CAD build for the part. Positions are in the model's coordinates, mm. Coordinates: 2 decimals unless noted, no trailing zeros. Write each loop counter-clockwise with the first axis right and the second up, starting at its lowest first coordinate (ties: lowest second). Pieces come first, ordered by that corner, then holes. Notation, with made-up numbers: (54, 62) - (112, 62) arc R8 ccw to (112, 77) - close; hole circle Ø9 at (19.25, 76). An arc over 180 degrees is marked (long way). Answer in a Markdown table with one row per item. Add a question column.
Q1. Band-saw the part on C-C (x = 116). List the corners of the cut face in (y, z).
Q2. Band-saw the part on B-B (y = 6). List the corners of the cut face in (x, z), and give its area (3 significant figures).
Q3. Pin check, flat tips, straight feed: pin 1 (3.5 mm diameter, centred on x = 4, y = 6, fed in from -Z); pin 2 (7 mm diameter, centred on x = 116, y = 6, fed in from +Z). Stop position of each tip, or through.
Q4. Band-saw the part on A-A (z = 1.35). List the corners of the cut face in (x, y).
Q5. Drill centre lines: line 1 along X through (y, z) = (6, 1.9); line 2 along X through (y, z) = (6.5, 4.2); line 3 along Y through (x, z) = (4, 0.85). Where is each one in solid material? Low to high. Write a range as from..to.
Q6. Band-saw the part on D-D (x = 89.5). List the corners of the cut face in (y, z), and give its area (3 significant figures).
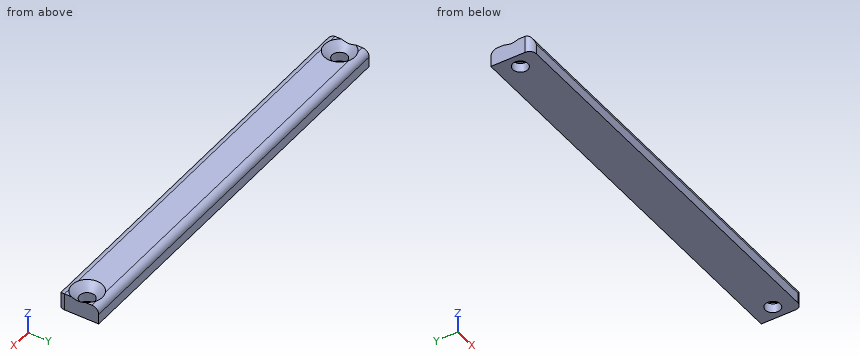
```python
from build123d import *

# Parameters (mm, degrees)
F0_W           = 120
F0_H           = 12
F1_DEPTH       = 5
F3_D           = 4.4
F3_DEPTH       = 18
F3_CSINK_D     = 8.96
F3_CSINK_ANGLE = 90
F3_TIP         = 1.3218933619
F4_T1_DEPTH    = 130
F4_T3_DEPTH    = 15


# Not quite as in the source:
# - a fillet or chamfer that OpenCascade refuses, or shapes differently, is made with other operations: its cross-section is extruded or revolved along the edge and cut away or added


with BuildPart() as f1:
    # F0 (on Top) → F1 (new body)
    with BuildSketch(Plane.XY):
        with Locations((60, 6)):
            Rectangle(F0_W, F0_H)
    extrude(amount=F1_DEPTH)

    # F3
    with Locations(Plane.XY.offset(5)):
        with Locations((4, 6), (116, 6)):
            CounterSinkHole(F3_D / 2, F3_CSINK_D / 2, depth=F3_DEPTH, counter_sink_angle=F3_CSINK_ANGLE)
            with Locations((0, 0, -(F3_DEPTH + F3_TIP / 2))):  # 118° drill point
                Cone(0, F3_D / 2, F3_TIP, mode=Mode.SUBTRACT)

    # F4: fillet of radius 2 on 4 edges, made by hand

    # F4_s2 → F4_t1 (cut)
    with BuildSketch(Plane.YZ.offset(-5)):
        with BuildLine():
            ThreePointArc((0, 3), (0.5857864376, 4.4142135624), (2, 5))
            Line((2, 5), (0, 5))
            Line((0, 5), (0, 3))
        make_face()
        with BuildLine():
            ThreePointArc((10, 5), (11.4142135624, 4.4142135624), (12, 3))
            Line((12, 3), (12, 5))
            Line((12, 5), (10, 5))
        make_face()
    extrude(amount=F4_T1_DEPTH, mode=Mode.SUBTRACT)

    # F4_s4 → F4_t3 (cut)
    with BuildSketch(Plane.XY.offset(-5)):
        with BuildLine():
            ThreePointArc((0, 2), (0.5857864376, 0.5857864376), (2, 0))
            Line((2, 0), (0, 0))
            Line((0, 0), (0, 2))
        make_face()
        with BuildLine():
            ThreePointArc((118, 0), (119.4142135624, 0.5857864376), (120, 2))
            Line((120, 2), (120, 0))
            Line((120, 0), (118, 0))
        make_face()
    extrude(amount=F4_T3_DEPTH, mode=Mode.SUBTRACT)


solid = f1.part
```
Checked values:
| question | item | result |
|---|---|---|
| 1 | outline | (0, 0) - (3.8, 0) - (3.8, 2.72) - (1.57, 4.95) arc R2 ccw to (0, 3) - close; (8.2, 0) - (12, 0) - (12, 3) arc R2 ccw to (10.43, 4.95) - (8.2, 2.72) - close |
| 2 | outline | (0, 0) - (1.8, 0) - (1.8, 2.72) - (0, 4.52) - close; (6.2, 0) - (113.8, 0) - (113.8, 2.72) - (111.52, 5) - (8.48, 5) - (6.2, 2.72) - close; (118.2, 0) - (120, 0) - (120, 4.52) - (118.2, 2.72) - close |
| 2 | area | 546 mm² |
| 3 | pin 1 | passes through |
| 3 | pin 2 | stops at z = 4.02 |
| 4 | outline | (0, 2) arc R2 ccw to (2, 0) - (118, 0) arc R2 ccw to (120, 2) - (120, 12) - (0, 12) - close; hole circle Ø4.4 at (4, 6); hole circle Ø4.4 at (116, 6) |
| 5 | line 1 | x = 0..1.8, 6.2..113.8, 118.2..120 |
| 5 | line 2 | x = 0..0.35, 7.65..112.35, 119.65..120 |
| 5 | line 3 | y = 0..3.8, 8.2..12 |
| 6 | outline | (0, 0) - (12, 0) - (12, 3) arc R2 ccw to (10, 5) - (2, 5) arc R2 ccw to (0, 3) - close |
| 6 | area | 58.3 mm² |
